Source: CAD feature listing. Evaluate the final solid. Frame: model axes, mm. A direction names the side the tool comes from. Give positions to 0.01 mm unless a question says otherwise; leave off trailing zeros. Loops run counter-clockwise (first coordinate to the right, second up) from the corner with the lowest first, then second, coordinate; pieces in that order, holes last.
from build123d import *

# Parameters (mm, degrees)
SKETCH_1_W                  = 80
SKETCH_1_H                  = 120
EXTRUDE_1_DEPTH             = 80
SKETCH_2_W                  = 19
SKETCH_2_H                  = 100
CUT_EXTRUDE_1_DEPTH         = 81
SKETCH_3_W                  = 19
SKETCH_3_H                  = 100
CUT_EXTRUDE_2_DEPTH         = 81
CUT_EXTRUDE_3_DEPTH         = 81
SKETCH_5_W                  = 34
SKETCH_5_H                  = 92
CUT_EXTRUDE_4_DEPTH         = 76
CUT_EXTRUDE_5_REACH         = 63
SKETCH_6_W                  = 49.5
SKETCH_6_H                  = 31.5
SKETCH_7_W                  = 49.5
SKETCH_7_H                  = 31.5
CUT_EXTRUDE_6_DEPTH         = 62
HOLE_WIZARD_1_8_1_8_5_D     = 1.8
HOLE_WIZARD_1_8_1_8_5_DEPTH = 4
HOLE_WIZARD_16_0_16_1_D     = 16
HOLE_WIZARD_1_8_1_8_4_D     = 1.8
HOLE_WIZARD_1_8_1_8_4_DEPTH = 4
HOLE_WIZARD_1_8_1_8_4_TIP   = 0.540774557
HOLE_WIZARD_1_8_1_8_3_D     = 1.8
HOLE_WIZARD_1_8_1_8_1_D     = 1.8
HOLE_WIZARD_1_8_1_8_1_DEPTH = 5.2
HOLE_WIZARD_1_8_1_8_1_TIP   = 0.540774557
HOLE_WIZARD_1_8_1_8_2_D     = 1.8
HOLE_WIZARD_1_8_1_8_2_DEPTH = 4
HOLE_WIZARD_1_8_1_8_2_TIP   = 0.540774557
EXTRUDE_2_DEPTH             = 80
SKETCH_21_R                 = 1.4
CUT_EXTRUDE_7_DEPTH         = 8
SKETCH_22_R                 = 1.4
CUT_EXTRUDE_8_DEPTH         = 8
SKETCH_23_R                 = 0.9
CUT_EXTRUDE_9_DEPTH         = 2


with BuildPart() as part:
    # 스케치1 → 보스-돌출1 (new body)
    with BuildSketch(Plane(origin=(0, 80, 0), x_dir=(1, 0, 0), z_dir=(0, 1, 0))):
        Rectangle(SKETCH_1_W, SKETCH_1_H)
    extrude(amount=-EXTRUDE_1_DEPTH)

    # 스케치2 → 컷-돌출1 (cut, through all)
    with BuildSketch(Plane.XZ):
        with Locations((-30.5, 10)):
            Rectangle(SKETCH_2_W, SKETCH_2_H)
    extrude(amount=-CUT_EXTRUDE_1_DEPTH, mode=Mode.SUBTRACT)

    # 스케치3 → 컷-돌출2 (cut, through all)
    with BuildSketch(Plane.XZ):
        with Locations((30.5, 10)):
            Rectangle(SKETCH_3_W, SKETCH_3_H)
    extrude(amount=-CUT_EXTRUDE_2_DEPTH, mode=Mode.SUBTRACT)

    # 스케치4 → 컷-돌출3 (cut, through all)
    with BuildSketch(Plane.XZ):
        with BuildLine():
            Line((-27.946377225, -60), (27.946377225, -60))
            ThreePointArc((27.946377225, -60), (0, -49), (-27.946377225, -60))
        make_face()
    extrude(amount=-CUT_EXTRUDE_3_DEPTH, mode=Mode.SUBTRACT)

    # 스케치5 → 컷-돌출4 (cut)
    with BuildSketch(Plane(origin=(0, 80, 0), x_dir=(-1, 0, 0), z_dir=(0, 1, 0))):
        with Locations((0, 10)):
            Rectangle(SKETCH_5_W, SKETCH_5_H)
    extrude(amount=-CUT_EXTRUDE_4_DEPTH, mode=Mode.SUBTRACT)

    # 스케치6 → 컷-돌출5 (cut, up to next)
    with BuildSketch(Plane(origin=(21, 0, 0), x_dir=(0, 0, -1), z_dir=(1, 0, 0)), mode=Mode.PRIVATE) as cut_extrude_5_sk1:
        with Locations((-10, 40)):
            Rectangle(SKETCH_6_W, SKETCH_6_H)
    cut_extrude_5_tool1 = extrude(cut_extrude_5_sk1.sketch, amount=-CUT_EXTRUDE_5_REACH, mode=Mode.PRIVATE) & part.part
    add(cut_extrude_5_tool1.solids().sort_by_distance((21, 40, 10))[0], mode=Mode.SUBTRACT)

    # 스케치7 → 컷-돌출6 (cut, through all)
    with BuildSketch(Plane.ZY.offset(21)):
        with Locations((8.5, 40)):
            Rectangle(SKETCH_7_W, SKETCH_7_H)
    extrude(amount=-CUT_EXTRUDE_6_DEPTH, mode=Mode.SUBTRACT)

    # Ø1.8 (1.8) 지름 구멍5
    with Locations(Plane.ZY.offset(21)):
        with Locations((10, 78)):
            Hole(HOLE_WIZARD_1_8_1_8_5_D / 2, depth=HOLE_WIZARD_1_8_1_8_5_DEPTH)

    # Ø16.0 (16) 지름 구멍1 (through all)
    with Locations(Plane(origin=(0, 0, 0), x_dir=(-1, 0, 0), z_dir=(0, -1, 0))):
        with Locations((0, -22)):
            Hole(HOLE_WIZARD_16_0_16_1_D / 2)

    # Ø1.8 (1.8) 지름 구멍4
    with Locations(Plane.ZY.offset(21)):
        with Locations((-38, 78), (-38, 40), (-38, 2), (10, 2)):
            Hole(HOLE_WIZARD_1_8_1_8_4_D / 2, depth=HOLE_WIZARD_1_8_1_8_4_DEPTH)
            with Locations((0, 0, -(HOLE_WIZARD_1_8_1_8_4_DEPTH + HOLE_WIZARD_1_8_1_8_4_TIP / 2))):  # 118° drill point
                Cone(0, HOLE_WIZARD_1_8_1_8_4_D / 2, HOLE_WIZARD_1_8_1_8_4_TIP, mode=Mode.SUBTRACT)

    # Ø1.8 (1.8) 지름 구멍3 (through all)
    with Locations(Plane(origin=(21, 0, 0), x_dir=(0, 0, -1), z_dir=(1, 0, 0))):
        with Locations((-10, 78)):
            Hole(HOLE_WIZARD_1_8_1_8_3_D / 2)

    # Ø1.8 (1.8) 지름 구멍1
    with Locations(Plane(origin=(0, 80, 0), x_dir=(1, 0, 0), z_dir=(0, 1, 0))):
        with Locations((33.973188612, 50), (-33.973188612, 50)):
            Hole(HOLE_WIZARD_1_8_1_8_1_D / 2, depth=HOLE_WIZARD_1_8_1_8_1_DEPTH)
            with Locations((0, 0, -(HOLE_WIZARD_1_8_1_8_1_DEPTH + HOLE_WIZARD_1_8_1_8_1_TIP / 2))):  # 118° drill point
                Cone(0, HOLE_WIZARD_1_8_1_8_1_D / 2, HOLE_WIZARD_1_8_1_8_1_TIP, mode=Mode.SUBTRACT)

    # Ø1.8 (1.8) 지름 구멍2
    with Locations(Plane(origin=(21, 0, 0), x_dir=(0, 0, -1), z_dir=(1, 0, 0))):
        with Locations((38, 78), (38, 40), (38, 2), (-10, 2)):
            Hole(HOLE_WIZARD_1_8_1_8_2_D / 2, depth=HOLE_WIZARD_1_8_1_8_2_DEPTH)
            with Locations((0, 0, -(HOLE_WIZARD_1_8_1_8_2_DEPTH + HOLE_WIZARD_1_8_1_8_2_TIP / 2))):  # 118° drill point
                Cone(0, HOLE_WIZARD_1_8_1_8_2_D / 2, HOLE_WIZARD_1_8_1_8_2_TIP, mode=Mode.SUBTRACT)

    # 스케치20 → 보스-돌출2 (add)
    with BuildSketch(Plane(origin=(0, 80, 0), x_dir=(1, 0, 0), z_dir=(0, 1, 0))):
        Polygon((40, -37.5), (36, -37.5), (36, -56), (-36, -56), (-36, -37.5), (-40, -37.5), (-40, -60), (40, -60), align=None)
    extrude(amount=-EXTRUDE_2_DEPTH)

    # 스케치21 → 컷-돌출7 (cut)
    with BuildSketch(Plane.ZY.offset(40)):
        with Locations((-45, 23.75)):
            Circle(SKETCH_21_R)
        with Locations((-45, 56.25)):
            Circle(SKETCH_21_R)
    extrude(amount=-CUT_EXTRUDE_7_DEPTH, mode=Mode.SUBTRACT)

    # 스케치22 → 컷-돌출8 (cut)
    with BuildSketch(Plane(origin=(40, 0, 0), x_dir=(0, 0, -1), z_dir=(1, 0, 0))):
        with Locations((45, 23.75)):
            Circle(SKETCH_22_R)
        with Locations((45, 56.25)):
            Circle(SKETCH_22_R)
    extrude(amount=-CUT_EXTRUDE_8_DEPTH, mode=Mode.SUBTRACT)

    # 스케치23 → 컷-돌출9 (cut)
    with BuildSketch(Plane(origin=(0, 80, 0), x_dir=(1, 0, 0), z_dir=(0, 1, 0))):
        with Locations((-38, -58)):
            Circle(SKETCH_23_R)
        with Locations((0, -58)):
            Circle(SKETCH_23_R)
        with Locations((38, -58)):
            Circle(SKETCH_23_R)
    extrude(amount=-CUT_EXTRUDE_9_DEPTH, mode=Mode.SUBTRACT)


solid = part.part
1) Cut plane B-B (x = 29.5). Return loops of the section in (y, z), and give its area (3 significant figures).
Checks:
outline: (0, -60) - (80, -60) - (80, -40) - (0, -40) - close; (0, 56) - (80, 56) - (80, 60) - (0, 60) - close
area: 1,920 mm2
2) Cut plane C-C (z = 4). Return loops of the section in (x, y).
Checks:
outline: (-21, 0) - (21, 0) - (21, 24.25) - (17, 24.25) - (17, 4) - (-17, 4) - (-17, 24.25) - (-21, 24.25) - close; (-21, 55.75) - (-17, 55.75) - (-17, 80) - (-21, 80) - close; (17, 55.75) - (21, 55.75) - (21, 80) - (17, 80) - close
3) Pull-direction query (Z, two-part tool) for faces 1 (the flat face through (40, 41, -50)), 2 (the flat face through (-17, 59, 9)), 3 (the flat face through (-34, 41, -60)); classes: released by +Z, released by -Z, zero draft, split by the parting line, or undercut.
Checks:
face 1: zero draft
face 2: undercut
face 3: released by -Z
4) Contact query for flat-ended pins moving along their axis: P1, Ø5, axis at y = 14, z = -5, coming from the +X side; P2, Ø1.4, axis at y = 56, z = -44.5, coming from the -X side; P3, Ø3, axis at y = 23.75, z = -45, coming from the -X side; P4, Ø1.1, axis at y = 2, z = -38, coming from the +X side. Output: stop coordinate, or through.
Checks:
P1: stops at x = 21
P2: stops at x = -32
P3: stops at x = -40
P4: stops at x = 16.79
5) Reachability of faces 4 (the flat face through (-21, 22, 7)), 5 (the flat face through (-32, 24, -45)), 6 (the flat face through (-31, 39, -40)), 7 (the flat face through (32, 24, -45)), 8 (the flat face through (-19, 55.75, 8)) from +Z, -Z, +X, -X, +Y, -Y: full face, straight path, thin tool, end or side. Return the list, or none.
Checks:
face 4: +Y, -Y
face 5: -X
face 6: -X, +Y, -Y
face 7: +X
face 8: +X, -X
6) Cut plane A-A (y = 16). Return loops of the section in (x, z).
Checks:
outline: (-40, -60) - (-27.95, -60) arc R41 cw to (27.95, -60) - (40, -60) - (40, -40) - (21, -40) - (21, 56) - (36, 56) - (36, 37.5) - (40, 37.5) - (40, 60) - (-40, 60) - (-40, 37.5) - (-36, 37.5) - (-36, 56) - (-21, 56) - (-21, -40) - (-40, -40) - close; hole (-17, -36) - (17, -36) - (17, 56) - (-17, 56) - close
7) Ray query, probe 1 along X at (y, z) = (79, 58); probe 2 along X at (y, z) = (67.5, 20); probe 3 along X at (y, z) = (53, 45.5). Return the intervals inside material, ascending.
Checks:
probe 1: x = -40 to -38.9, -37.1 to -0.9, 0.9 to 37.1, 38.9 to 40
probe 2: x = -21 to -17, 17 to 21
probe 3: x = -40 to -36, -21 to -17, 17 to 21, 36 to 40
